Can you work these out from the model? Positions are in its coordinate system, mm. Face numbers are marked on the shaded views. Give positions to 0.01 mm unless a question says otherwise; leave off trailing zeros. Write each loop counter-clockwise with the first axis right and the second up, starting at its lowest first coordinate (ties: lowest second). Pieces come first, ordered by that corner, then holes.
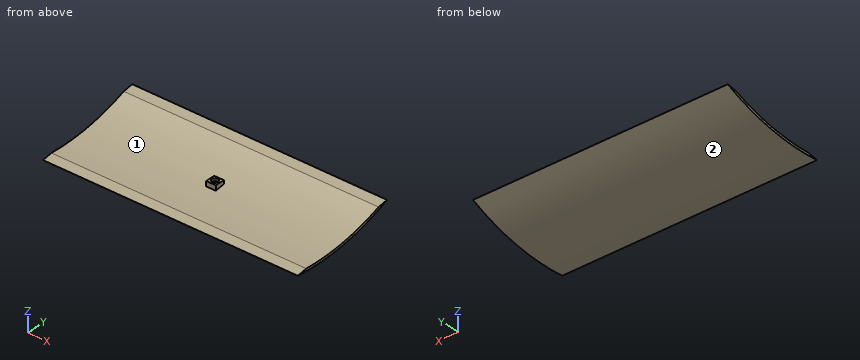
```python
from build123d import *

# Parameters (mm, degrees)
BOSS_EXTRUDE2_DEPTH      = 150
BOSS_EXTRUDE2_DEPTH_BACK = 50
BOSS_EXTRUDE3_REACH      = 387.24
BOSS_EXTRUDE3_END_RADIUS = 160.09
BOSS_EXTRUDE3_START      = -155
SKETCH2_W                = 7.5
SKETCH2_H                = 7.5
SKETCH3_R                = 2.5
CUT_EXTRUDE1_DEPTH       = 2


with BuildPart() as part:
    # Sketch1 → Boss-Extrude2 (new, two sides: drawn at the far end of the back side and taken through both)
    with BuildSketch(Plane(origin=(0, 0, 0), x_dir=(0, 0, -1), z_dir=(1, 0, 0)).offset(-BOSS_EXTRUDE2_DEPTH_BACK)):
        with BuildLine():
            Line((148.248037227, 65.318599636), (149.44212598, 57.409573092))
            ThreePointArc((149.44212598, 57.409573092), (158.29603806, 23.899214101), (159.729912673, -10.731407065))
            Line((159.729912673, -10.731407065), (160.924001426, -18.640433609))
            ThreePointArc((160.924001426, -18.640433609), (160.184634678, 24.18435058), (148.248037227, 65.318599636))
        make_face()
    extrude(amount=BOSS_EXTRUDE2_DEPTH + BOSS_EXTRUDE2_DEPTH_BACK)

    # Boss-Extrude3: up to this cylinder (the profile starts inside it)
    boss_extrude3_end = Plane(origin=(50, 0, 0), z_dir=(1, 0, 0)) * Cylinder(BOSS_EXTRUDE3_END_RADIUS, 1095.66, mode=Mode.PRIVATE)
    # Sketch2 → Boss-Extrude3 (add, up to the surface)
    with BuildSketch(Plane.XY.offset(BOSS_EXTRUDE3_START), mode=Mode.PRIVATE) as boss_extrude3_sk1:
        with Locations((50, 23.339083013)):
            Rectangle(SKETCH2_W, SKETCH2_H)
    boss_extrude3_tool1 = extrude(boss_extrude3_sk1.sketch, amount=-BOSS_EXTRUDE3_REACH, mode=Mode.PRIVATE) & boss_extrude3_end
    add(boss_extrude3_tool1.solids().sort_by_distance((50, 23.339083, -155))[0])

    # Sketch3 → Cut-Extrude1 (cut)
    with BuildSketch(Plane.XY.offset(-155)):
        with Locations((50, 23.339083013)):
            Circle(SKETCH3_R)
    extrude(amount=-CUT_EXTRUDE1_DEPTH, mode=Mode.SUBTRACT)


solid = part.part
```
1) Please list where these lines run through material, in increasing order: L1, parallel to Z at x = 23.5, y = 2.5; L2, parallel to Z at x = 10.5, y = 41.
Values follow:
L1: z = -161.98 to -160.07
L2: z = -156.73 to -154.75
2) For pin 1 Ø1.2 at (y, z) = (22.5, -156.5) entering from -X; pin 2 Ø5.5 at (x, y) = (49.5, 22) entering from +Z; pin 3 Ø10 at (x, y) = (-7.5, 29) entering from -Z; pin 4 Ø1 at (y, z) = (19, -157) entering from -X, each with a flat end and sliding along its axis, tell me the tip position at first contact or that it passes through.
Values follow:
pin 1: stops at x = 46.25
pin 2: stops at z = -155
pin 3: stops at z = -160.21
pin 4: passes through
3) Suppose I cut it at C-C on x = -4. Write out the boundary of the cut face in (y, z), plus the area to 3 significant figures.
Values follow:
outline: (-18.64, -160.92) arc R162 ccw to (65.32, -148.25) - (57.41, -149.44) arc R160.09 cw to (-10.73, -159.73) - close
area: 149 mm2
4) If we mould it in two halves opening along Y, with no side actions, what happens to the marked faces 1 and 2? For each: +Y half, -Y half, draft (parallel to the pull), parting line (faces both ways), or undercut.
Values follow:
face 1: undercut
face 2: parting line
5) Suppose I cut it at A-A on x = 50. Write out the boundary of the cut face in (y, z).
Values follow:
outline: (-18.64, -160.92) arc R162 ccw to (65.32, -148.25) - (57.41, -149.44) arc R160.09 cw to (27.09, -157.78) - (27.09, -155) - (25.84, -155) - (25.84, -157) - (20.84, -157) - (20.84, -155) - (19.59, -155) - (19.59, -158.89) arc R160.09 cw to (-10.73, -159.73) - close
